Print and shaded views of the part. All mm, measured from the part's lowest x, y and z. A direction names the side the tool comes from. Coordinates: 2 decimals unless noted, no trailing zeros. Order: outer loops, then holes, each group sorted by start corner. A loop starts at its lowest first (then second) coordinate and runs counter-clockwise, first axis right, second up. Notation, with made-up numbers: M -17,51 L -11,51 A12 ccw -11,74 Z; hole C -22.5,-9 d7. An arc over 180 degrees is marked long. Return JSON: item names as keys, results as strings.
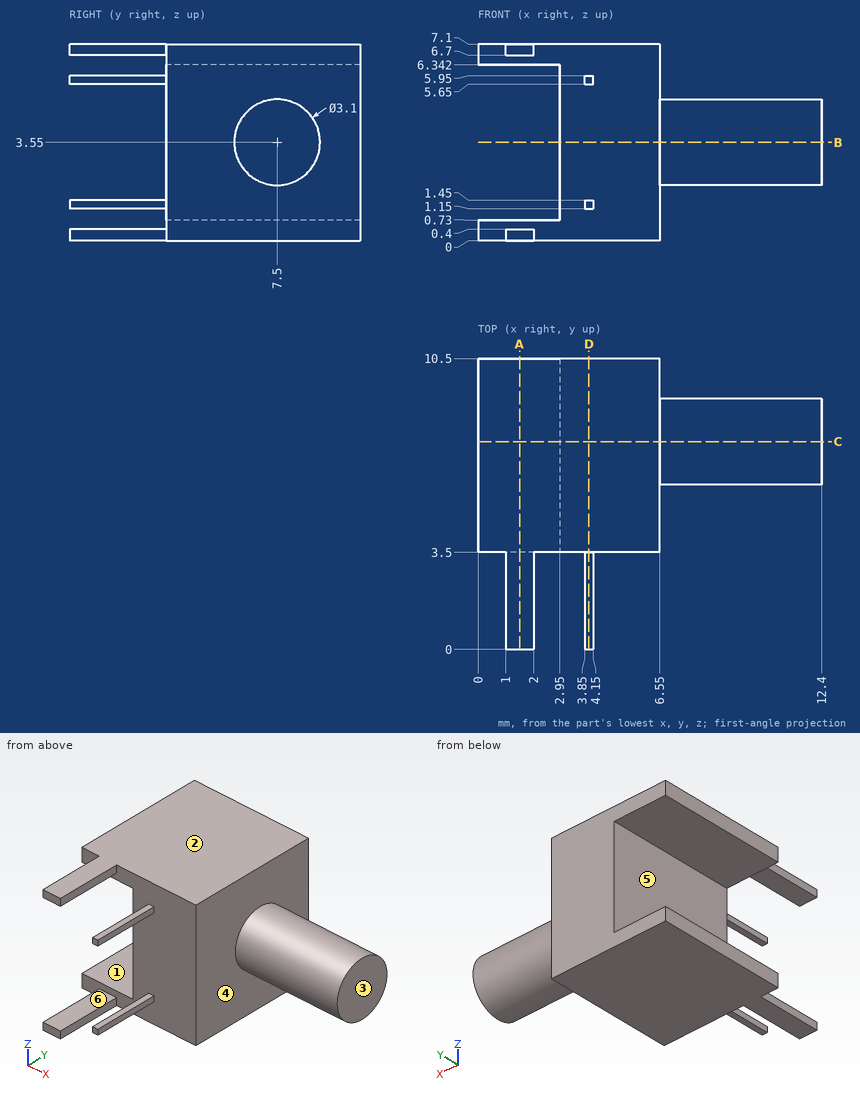
Item 1: Pull direction Z, two halves, no side cores. Call the marked faces 1, 2 and 3: +Z half, -Z half, draft (parallel to the pull), parting line (faces both ways), or undercut.
Check result:
{"face 1": "undercut", "face 2": "+Z half", "face 3": "draft"}
Item 2: Saw through at C-C (y = 7.5). Write the cut outline in (x, z).
Check result:
{"outline": "M 0,0 L 6.55,0 L 6.55,2 L 12.4,2 L 12.4,5.1 L 6.55,5.1 L 6.55,7.1 L 0,7.1 L 0,6.34 L 2.95,6.34 L 2.95,0.73 L 0,0.73 Z"}
Item 3: Wall check: line 1 (Z direction, x = 1.5, y = 4); line 2 (X direction, y = 9.5, z = 5.5); line 3 (X direction, y = 9.75, z = 0.5). Give the ranges that are in metal, low to high.
Check result:
{"line 1": "z = 0 to 0.73, 6.34 to 7.1", "line 2": "x = 2.95 to 6.55", "line 3": "x = 0 to 6.55"}
Item 4: Saw through at D-D (x = 4). Write the cut outline in (y, z).
Check result:
{"outline": "M 0,1.15 L 3.5,1.15 L 3.5,0 L 10.5,0 L 10.5,7.1 L 3.5,7.1 L 3.5,5.95 L 0,5.95 L 0,5.65 L 3.5,5.65 L 3.5,1.45 L 0,1.45 Z"}
Item 5: Saw through at B-B (z = 3.55). Write the cut outline in (x, y).
Check result:
{"outline": "M 2.95,3.5 L 6.55,3.5 L 6.55,5.95 L 12.4,5.95 L 12.4,9.05 L 6.55,9.05 L 6.55,10.5 L 2.95,10.5 Z"}
Item 6: Drop flat-ended pins along their axis: pin 1 Ø3 at (x, z) = (10, 5) entering from -Y; pin 2 Ø1.7 at (y, z) = (5.5, 4.5) entering from -X; pin 3 Ø3 at (y, z) = (3.5, 6) entering from +X. Give the stop position or say it passes through.
Check result:
{"pin 1": "stops at y = 5.95", "pin 2": "stops at x = 2.95", "pin 3": "stops at x = 6.55"}
Item 7: Saw through at A-A (x = 1.5). Write the cut outline in (y, z).
Check result:
{"outline": "M 0,0 L 10.5,0 L 10.5,0.73 L 3.5,0.73 L 3.5,0.4 L 0,0.4 Z; M 0,6.7 L 3.5,6.7 L 3.5,6.34 L 10.5,6.34 L 10.5,7.1 L 0,7.1 Z"}
Item 8: 3-axis set-ups, long thin cutter, end or side, ignore diameter. For the marked faces 4, 5 and 6: which of +Z, -Z, +X, -X, +Y, -Y reach the whole face in a straight line?
Check result:
{"face 4": "+X", "face 5": "-X, +Y, -Y", "face 6": "+X, -X, -Y"}
